Geometry: see drawing. Coordinates: mm, zero at the bounding-box minimum. A direction names the side the tool comes from. Round coordinates to 2 decimals unless told otherwise and drop trailing zeros. Write each loop counter-clockwise with the first axis right and the second up, starting at its lowest first coordinate (ties: lowest second). Pieces come first, ordered by that corner, then holes. Notation, with made-up numbers: (-13.75, -29) -> (2.25, -29) arc R12 ccw to (2.25, -25) -> close; hole circle Ø8 at (-17, 50). An arc over 180 degrees is marked (long way). Use CSV: the item, a comma, the result in double quotes.
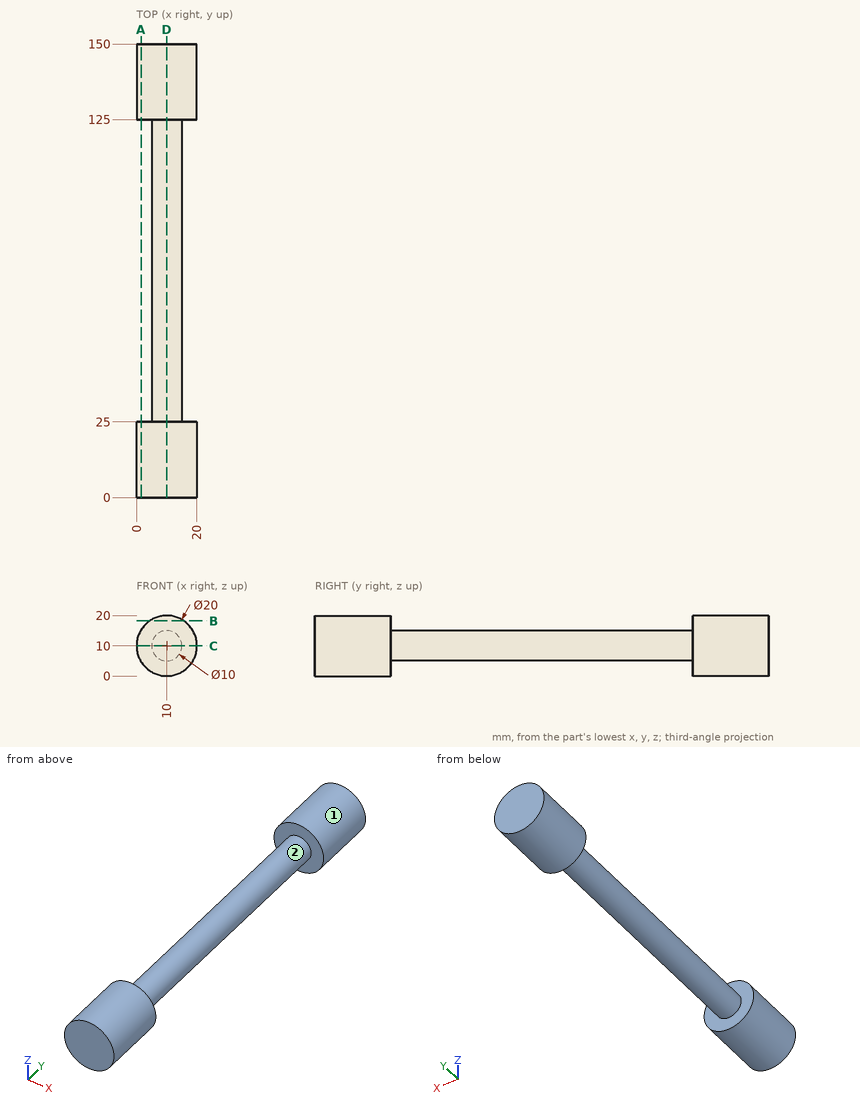
Item 1: Section query C-C on z = 10. Return the cut outline in (x, y), plus the area to 3 significant figures.
Worked answers:
outline,"(0, 0) -> (20, 0) -> (20, 25) -> (15, 25) -> (15, 125) -> (20, 125) -> (20, 150) -> (0, 150) -> (0, 125) -> (5, 125) -> (5, 25) -> (0, 25) -> close"
area,"2,000 mm²"
Item 2: Section query D-D on x = 10. Return the cut outline in (y, z).
Worked answers:
outline,"(0, 0) -> (25, 0) -> (25, 5) -> (125, 5) -> (125, 0) -> (150, 0) -> (150, 20) -> (125, 20) -> (125, 15) -> (25, 15) -> (25, 20) -> (0, 20) -> close"
Item 3: First-contact query: pin 1 Ø1.5 at (x, y) = (13, 42) entering from +Z; pin 2 Ø4 at (y, z) = (42, 9) entering from -X; pin 3 Ø1 at (x, y) = (13.5, 45) entering from +Z. Flat tips, straight axial feed; report the tip coordinate or a pass-through.
Worked answers:
pin 1,"stops at z = 14.47"
pin 2,"stops at x = 5"
pin 3,"stops at z = 14"
Item 4: Line query: line 1 (Y direction, x = 2.5, z = 5); line 2 (X direction, y = 82, z = 9.75); line 3 (X direction, y = 115, z = 8). Output: solid intervals per line, ascending.
Worked answers:
line 1,"y = 0 to 25, 125 to 150"
line 2,"x = 5.01 to 14.99"
line 3,"x = 5.42 to 14.58"
Item 5: Section query A-A on x = 1.5. Return the cut outline in (y, z).
Worked answers:
outline,"(0, 4.73) -> (25, 4.73) -> (25, 15.27) -> (0, 15.27) -> close; (125, 4.73) -> (150, 4.73) -> (150, 15.27) -> (125, 15.27) -> close"
Item 6: Section query B-B on z = 18.25. Return the cut outline in (x, y), plus the area to 3 significant figures.
Worked answers:
outline,"(4.35, 0) -> (15.65, 0) -> (15.65, 25) -> (4.35, 25) -> close; (4.35, 125) -> (15.65, 125) -> (15.65, 150) -> (4.35, 150) -> close"
area,"565 mm²"
Item 7: Set-up query: the marked faces 1 and 2. Return all of +Z, -Z, +X, -X, +Y, -Y with unobstructed straight access to the full face (end or side cutting, diameter ignored); none if empty.
Worked answers:
face 1,"+Y, -Y"
face 2,"none"
